from build123d import *

# Parameters (mm, degrees)
F0_R           = 10
F1_DEPTH       = 25
F3_D           = 10
F3_DEPTH       = 15
F3_CSINK_D     = 16
F3_CSINK_ANGLE = 90
F5_D           = 10
F5_DEPTH       = 15
F5_CSINK_D     = 16
F5_CSINK_ANGLE = 90


with BuildPart() as f1:
    # F0 (on Top) → F1 (new body)
    with BuildSketch(Plane.XY):
        Circle(F0_R)
    extrude(amount=F1_DEPTH)

    # F3
    with Locations(Plane.XY.offset(25)):
        with Locations((0, 0)):
            CounterSinkHole(F3_D / 2, F3_CSINK_D / 2, depth=F3_DEPTH, counter_sink_angle=F3_CSINK_ANGLE)

    # F5
    with Locations(Plane(origin=(0, 0, 0), x_dir=(1, 0, 0), z_dir=(0, 0, -1))):
        with Locations((0, 0)):
            CounterSinkHole(F5_D / 2, F5_CSINK_D / 2, depth=F5_DEPTH, counter_sink_angle=F5_CSINK_ANGLE)


solid = f1.part
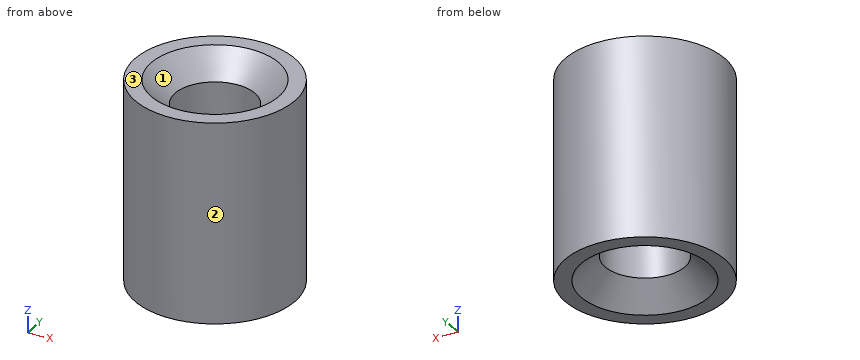
CAD build for the part. Positions are in the model's coordinates, mm. Face numbers are marked on the shaded views. Coordinates: 2 decimals unless noted, no trailing zeros. Write each loop counter-clockwise with the first axis right and the second up, starting at its lowest first coordinate (ties: lowest second). Pieces come first, ordered by that corner, then holes. Notation, with made-up numbers: (-23.75, 27) - (26.25, 27) arc R16 cw to (26.25, 51) - close; hole circle Ø2 at (18, 54.25). An arc over 180 degrees is marked (long way). Use a Markdown table: item, result. Add a question column.
Item 1: Band-saw the part on D-D, the plane z = 8. Give the cut face in (x, y).
Item 2: Drill centre lines: L1, parallel to Y at x = 0, z = 17.5; L2, parallel to X at y = 0.5, z = 17.5; L3, parallel to Y at x = -0.75, z = 6.5. Where is each one in solid material? Low to high. Write a range as from..to.
Item 3: Band-saw the part on C-C, the plane z = 23. Give the cut face in (x, y).
Item 4: Flat gauge pins, fed straight in: pin 1 (2 mm diameter, centred on x = 3, y = 5, fed in from -Z); pin 2 (2 mm diameter, centred on x = -6, y = 0.5, fed in from +Z); pin 3 (2 mm diameter, centred on x = 7, y = -4.5, fed in from -Z); pin 4 (4 mm diameter, centred on y = 3.5, z = 22, fed in from -X). Where does each tip first touch, or does it go through?
Item 5: Band-saw the part on A-A, the plane y = 0. Give the cut face in (x, z), and give its area (3 significant figures).
Item 6: Mould opens along X. For the marked faces 1, 2 and 3 say: pulls with the +X half, pulls with the -X half, needs draft (parallel to the pull), parting line crosses it, or undercut.
Numbers:
| question | item | result |
|---|---|---|
| 1 | outline | circle Ø20 at (0, 0); hole circle Ø10 at (0, 0) |
| 2 | L1 | -10..-5, 5..10 |
| 2 | L2 | -9.99..-4.97, 4.97..9.99 |
| 2 | L3 | -9.97..-4.94, 4.94..9.97 |
| 3 | outline | circle Ø20 at (0, 0); hole circle Ø12 at (0, 0) |
| 4 | pin 1 | z = 1.17 |
| 4 | pin 2 | z = 24.02 |
| 4 | pin 3 | z = 0 |
| 4 | pin 4 | x = -9.89 |
| 5 | outline | (-10, 0) - (-8, 0) - (-5, 3) - (-5, 22) - (-8, 25) - (-10, 25) - close; (5, 3) - (8, 0) - (10, 0) - (10, 25) - (8, 25) - (5, 22) - close |
| 5 | area | 232 mm2 |
| 6 | face 1 | undercut |
| 6 | face 2 | parting line crosses it |
| 6 | face 3 | needs draft |
